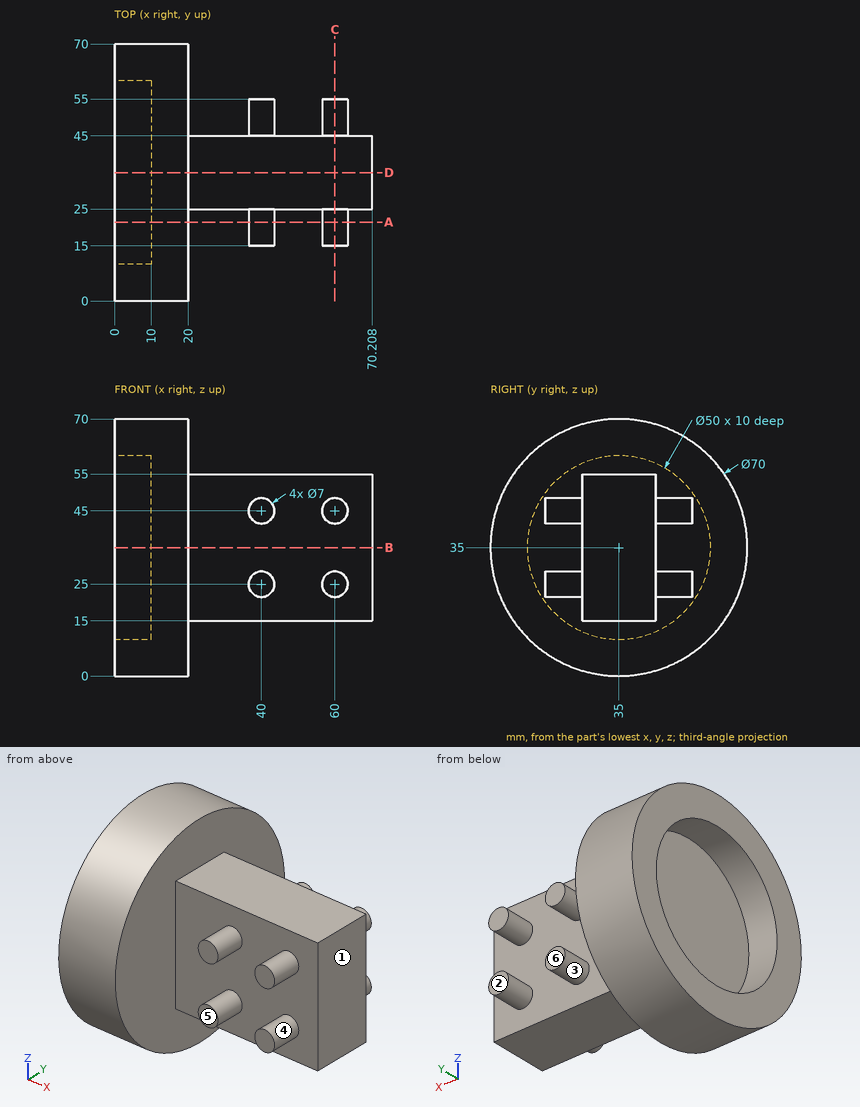
Input: dimensioned drawing with shaded views. Units: mm. Origin: part minimum x, y, z. A direction names the side the tool comes from. Give positions to 0.01 mm unless a question says otherwise; leave off trailing zeros. Loops run counter-clockwise (first coordinate to the right, second up) from the corner with the lowest first, then second, coordinate; pieces in that order, holes last. Notation, with made-up numbers: (88, 41) -> (125, 41) arc R17 ccw to (125, 55) -> close; hole circle Ø1 at (16, 57.25). An arc over 180 degrees is marked (long way). Use a Markdown table: item, result. Add a question column.
1) Section query B-B, the plane z = 35. Return the cut outline in (x, y), then the cut area to 3 significant figures.
2) Section query C-C, the plane x = 60. Return the cut outline in (y, z), then the cut area to 3 significant figures.
3) First-contact query: pin 1 (6 mm diameter, centred on y = 14, z = 9.5, fed in from -X); pin 2 (7.5 mm diameter, centred on x = 59, z = 25, fed in from +Y); pin 3 (25 mm diameter, centred on y = 42.5, z = 35.5, fed in from -X); pin 4 (2 mm diameter, centred on x = 20, y = 45.5, fed in from -Z). Flat tips, straight axial feed; report the tip coordinate or a pass-through.
4) Line query: line 1 along Y through (x, z) = (7, 35); line 2 along X through (y, z) = (61.5, 16); line 3 along X through (y, z) = (28.5, 36). Output: solid intervals per line, ascending. Write a range as [from, to].
5) Pull-direction query (X, two-part tool) for the marked faces 1, 2 and 3; classes: +X half, -X half, draft (parallel to the pull), parting line (faces both ways), or undercut.
6) Reachability of the marked faces 4, 5 and 6 from +Z, -Z, +X, -X, +Y, -Y: full face, straight path, thin tool, end or side. Return the list, or none.
7) Section query A-A, the plane y = 21.5. Return the cut outline in (x, z), then the cut area to 4 significant figures.
8) Section query D-D, the plane y = 35. Return the cut outline in (x, z), then the cut area to 3 significant figures.
Numbers:
| question | item | result |
|---|---|---|
| 1 | outline | (0, 0) -> (20, 0) -> (20, 25) -> (70.21, 25) -> (70.21, 45) -> (20, 45) -> (20, 70) -> (0, 70) -> (0, 60) -> (10, 60) -> (10, 10) -> (0, 10) -> close |
| 1 | area | 1,900 mm2 |
| 2 | outline | (15, 21.5) -> (25, 21.5) -> (25, 15) -> (45, 15) -> (45, 21.5) -> (55, 21.5) -> (55, 28.5) -> (45, 28.5) -> (45, 41.5) -> (55, 41.5) -> (55, 48.5) -> (45, 48.5) -> (45, 55) -> (25, 55) -> (25, 48.5) -> (15, 48.5) -> (15, 41.5) -> (25, 41.5) -> (25, 28.5) -> (15, 28.5) -> close |
| 2 | area | 1,080 mm2 |
| 3 | pin 1 | stops at x = 0 |
| 3 | pin 2 | stops at y = 55 |
| 3 | pin 3 | stops at x = 10 |
| 3 | pin 4 | stops at z = 1.31 |
| 4 | line 1 | y = [0, 10], [60, 70] |
| 4 | line 2 | x = [0, 20] |
| 4 | line 3 | x = [10, 70.21] |
| 5 | face 1 | +X half |
| 5 | face 2 | draft |
| 5 | face 3 | undercut |
| 6 | face 4 | -Y |
| 6 | face 5 | +Z, -Z, +X, -Y |
| 6 | face 6 | +Z, -Z, +X, +Y |
| 7 | outline | (0, 2.71) -> (20, 2.71) -> (20, 67.29) -> (0, 67.29) -> (0, 56.04) -> (10, 56.04) -> (10, 13.96) -> (0, 13.96) -> close; circle Ø7 at (40, 25); circle Ø7 at (40, 45); circle Ø7 at (60, 25); circle Ø7 at (60, 45) |
| 7 | area | 1,025 mm2 |
| 8 | outline | (0, 0) -> (20, 0) -> (20, 15) -> (70.21, 15) -> (70.21, 55) -> (20, 55) -> (20, 70) -> (0, 70) -> (0, 60) -> (10, 60) -> (10, 10) -> (0, 10) -> close |
| 8 | area | 2,910 mm2 |
